For this review, use the dimensioned drawing (mm, ordinates from the lowest corner) and the shaded views. A direction names the side the tool comes from. Coordinates: 2 decimals unless noted, no trailing zeros. Order: outer loops, then holes, each group sorted by start corner. A loop starts at its lowest first (then second) coordinate and runs counter-clockwise, first axis right, second up. Notation, with made-up numbers: M 17,79.5 L 52,79.5 A21 ccw 52,98.5 Z; hole C -32.5,41 d3. An arc over 180 degrees is marked long. Answer in a Markdown table with one row per item.
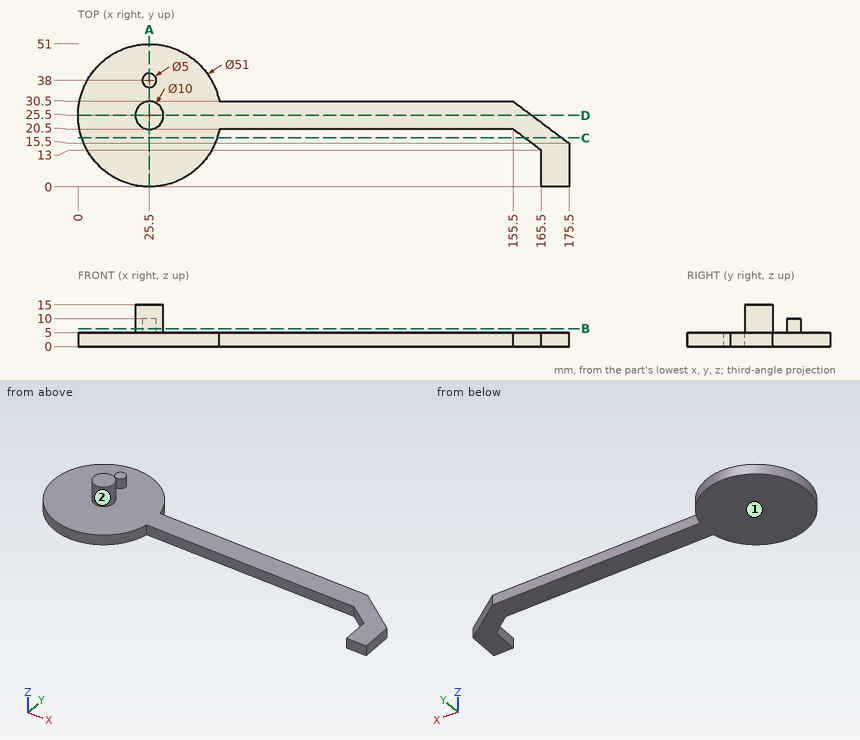
(1) For line 1 along Z through (x, y) = (19.5, 25); line 2 along X through (y, z) = (8, 1.5); line 3 along X through (y, z) = (8.5, 1), list the stretches that pass through material, from the lowest coordinate up. Write a range as from..to.
Return value:
| item | result |
|---|---|
| line 1 | z = 0..5 |
| line 2 | x = 6.95..44.05, 165.5..175.5 |
| line 3 | x = 6.49..44.51, 165.5..175.5 |
(2) Add section D-D, the plane y = 25.5. Give the boundary of the cut face in (x, z), and give its area (3 significant figures).
Return value:
| item | result |
|---|---|
| outline | M 0,0 L 162.17,0 L 162.17,5 L 30.5,5 L 30.5,15 L 20.5,15 L 20.5,5 L 0,5 Z |
| area | 911 mm2 |
(3) For the marked faces 1 and 2, list the 3-axis set-ups (+Z, -Z, +X, -X, +Y, -Y) from which the entire face can be reached by the end or side of a thin tool; tool diameter is ignored.
Return value:
| item | result |
|---|---|
| face 1 | -Z, +X, -X, +Y, -Y |
| face 2 | +Z |
(4) Insertion check: pin 1 Ø1.5 at (y, z) = (4.5, 2) entering from -X; pin 2 Ø1.5 at (x, z) = (123.5, 3) entering from +Y; pin 3 Ø5 at (y, z) = (36, 1.5) entering from -X; pin 4 Ø8 at (x, y) = (36, 17.5) entering from -Z. Each pin has a flat end and moves straight along its axis. Give the tip position at first contact, or say it passes through.
Return value:
| item | result |
|---|---|
| pin 1 | stops at x = 10 |
| pin 2 | stops at y = 30.5 |
| pin 3 | stops at x = 1.29 |
| pin 4 | stops at z = 0 |
(5) Add section B-B, the plane z = 6.5. Give the boundary of the cut face in (x, y).
Return value:
| item | result |
|---|---|
| outline | C 25.5,25.5 d10; C 25.5,38 d5 |
(6) Add section A-A, the plane x = 25.5. Give the boundary of the cut face in (y, z).
Return value:
| item | result |
|---|---|
| outline | M 0,0 L 51,0 L 51,5 L 40.5,5 L 40.5,10 L 35.5,10 L 35.5,5 L 30.5,5 L 30.5,15 L 20.5,15 L 20.5,5 L 0,5 Z |
(7) Add section C-C, the plane y = 17.5. Give the boundary of the cut face in (x, z), and give its area (3 significant figures).
Return value:
| item | result |
|---|---|
| outline | M 1.29,0 L 49.71,0 L 49.71,5 L 1.29,5 Z; M 159.5,0 L 172.83,0 L 172.83,5 L 159.5,5 Z |
| area | 309 mm2 |
